The listing builds one solid part. Answer for the finished solid, in the listing's coordinates (mm). A direction names the side the tool comes from. Give positions to 0.01 mm unless a question says otherwise; leave off trailing zeros. Order: outer loops, then holes, each group sorted by start corner. A loop starts at its lowest first (then second) coordinate and runs counter-clockwise, first axis right, second up.
```python
from build123d import *

# Parameters (mm, degrees)
CROQUIS1_W              = 200
CROQUIS1_H              = 150
SALIENTE_EXTRUIR1_DEPTH = 200
VACIADO1_T              = -3
CROQUIS2_R              = 12.7
SALIENTE_EXTRUIR2_DEPTH = 3
CROQUIS4_R              = 15
SALIENTE_EXTRUIR3_DEPTH = 90
CROQUIS6_R              = 10
SALIENTE_EXTRUIR4_DEPTH = 90
SALIENTE_EXTRUIR5_DEPTH = 90


with BuildPart() as part:
    # Croquis1 → Saliente-Extruir1 (new body)
    with BuildSketch(Plane.XY):
        with Locations((100, 75)):
            Rectangle(CROQUIS1_W, CROQUIS1_H)
    extrude(amount=SALIENTE_EXTRUIR1_DEPTH)

    # Vaciado1
    vaciado1_openings = [part.faces().sort_by_distance(p)[0] for p in [
        (100, 75, 200),
    ]]
    offset(amount=VACIADO1_T, openings=vaciado1_openings, kind=Kind.INTERSECTION)

    # Croquis2 → Saliente-Extruir2 (add)
    with BuildSketch(Plane(origin=(0, 150, 0), x_dir=(1, 0, 0), z_dir=(0, 1, 0))):
        with BuildLine():
            Line((150, 0), (50, 0))
            Line((50, 0), (80.716237825, -439.262665799))
            ThreePointArc((80.716237825, -439.262665799), (100, -457.245064944), (119.283762175, -439.262665799))
            Line((119.283762175, -439.262665799), (150, 0))
        make_face()
        with Locations(Location((100, -437.914213787, 0), (0, 0, 90))):
            Circle(CROQUIS2_R, mode=Mode.SUBTRACT)
    saliente_extruir2 = extrude(amount=SALIENTE_EXTRUIR2_DEPTH)

    # Simetría1: Saliente-Extruir2 across plane
    add(saliente_extruir2.mirror(Plane(origin=(0, 75, 0), x_dir=(0, 0, 1), z_dir=(0, -1, 0))))

    # Croquis4 → Saliente-Extruir3 (add)
    with BuildSketch(Plane(origin=(0, 3, 0), x_dir=(1, 0, 0), z_dir=(0, 1, 0))):
        with Locations(Location((100, -95, 0), (0, 0, 90))):
            Circle(CROQUIS4_R)
    extrude(amount=SALIENTE_EXTRUIR3_DEPTH)

    # Croquis6 → Saliente-Extruir4 (add)
    with BuildSketch(Plane(origin=(0, 0, 0), x_dir=(1, 0, 0), z_dir=(0, 1, 0))):
        with Locations(Location((100, -230, 0), (0, 0, 90))):
            Circle(CROQUIS6_R)
    extrude(amount=SALIENTE_EXTRUIR4_DEPTH)

    # Croquis7 → Saliente-Extruir5 (add)
    with BuildSketch(Plane(origin=(0, 3, 0), x_dir=(1, 0, 0), z_dir=(0, 1, 0))):
        Polygon((146.429598438, -170), (163.429598438, -170), (163.429598438, -200), align=None)
    extrude(amount=SALIENTE_EXTRUIR5_DEPTH)


solid = part.part
```
1) Given P1, Ø8, axis at x = 128, y = 69.5, coming from the +Z side; P2, Ø19, axis at x = 164.5, z = 106.5, coming from the +Y side; P3, Ø19, axis at x = 177.5, z = 55, coming from the -Y side, each flat-ended and moving along its own axis, determine where each tip first touches the part or whether it passes through.
Geometry says:
P1: stops at z = 3
P2: stops at y = 150
P3: stops at y = 0
2) Find section B-B (y = 78). Write down the section's boundary in (x, z).
Geometry says:
outline: (0, 0) - (200, 0) - (200, 200) - (197, 200) - (197, 3) - (3, 3) - (3, 200) - (0, 200) - close; circle Ø30 at (100, 95); circle Ø20 at (100, 230); (146.43, 170) - (163.43, 170) - (163.43, 200) - close
3) A tool of negligible diameter and unlimited length cuts with its end or side. For faces 4 (the flat face through (65.143, -1.479, 216.556)), 5 (the flat face through (155, 47, 170)), 6 (the flat face through (157, 93, 181)), from which of +Z, -Z, +X, -X, +Y, -Y can it reach the whole face along a straight path? Write none if from no direction.
Geometry says:
face 4: +Z, -X, -Y
face 5: none
face 6: +Z
4) For a pull along Y with two mould halves and no side action, classify faces 1 (the flat face through (99, 0, 298)), 2 (the flat face through (134.427, -1.479, 222.706)), 3 (the flat face through (99, 153, 175)) as +Y half, -Y half, draft (parallel to the pull), parting line (faces both ways), or undercut.
Geometry says:
face 1: undercut
face 2: draft
face 3: +Y half
5) Find section C-C (z = 346). Write down the section's boundary in (x, y), then the cut area to 3 significant figures.
Geometry says:
outline: (74.19, -3) - (125.81, -3) - (125.81, 0) - (74.19, 0) - close; (74.19, 150) - (125.81, 150) - (125.81, 153) - (74.19, 153) - close
area: 310 mm2
6) Find section A-A (x = 100). Write down the section's boundary in (y, z).
Geometry says:
outline: (-3, 0) - (153, 0) - (153, 425.21) - (150, 425.21) - (150, 200) - (147, 200) - (147, 3) - (3, 3) - (3, 80) - (93, 80) - (93, 110) - (3, 110) - (3, 200) - (0, 200) - (0, 220) - (90, 220) - (90, 240) - (0, 240) - (0, 425.21) - (-3, 425.21) - close; (-3, 450.61) - (0, 450.61) - (0, 457.25) - (-3, 457.25) - close; (150, 450.61) - (153, 450.61) - (153, 457.25) - (150, 457.25) - close
7) Straight lines are drawn through the part: probe 1 along Y at (x, z) = (107, 323); probe 2 along Z at (x, y) = (100, -0.75); probe 3 along Y at (x, z) = (149.5, 25). For each, find the intervals that lie inside material, in ascending order.
Geometry says:
probe 1: y = -3 to 0, 150 to 153
probe 2: z = 0 to 425.21, 450.61 to 457.25
probe 3: y = 0 to 3, 147 to 150
8) Find section D-D (y = 107.5). Write down the section's boundary in (x, z).
Geometry says:
outline: (0, 0) - (200, 0) - (200, 200) - (197, 200) - (197, 3) - (3, 3) - (3, 200) - (0, 200) - close
